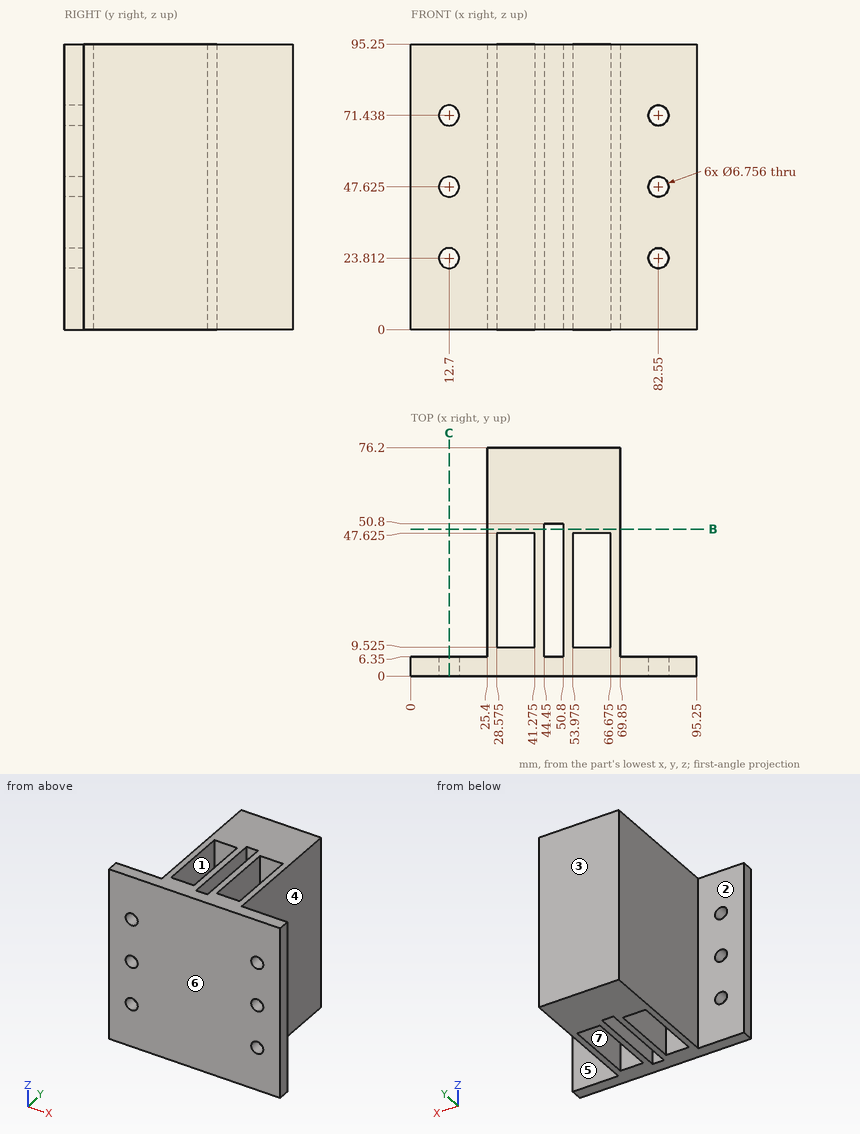
Here's the drawing with two shaded views (mm, measured from the low corner). I have some questions. A direction names the side the tool comes from. Give positions to 0.01 mm unless a question says otherwise; leave off trailing zeros. Order: outer loops, then holes, each group sorted by start corner. A loop starts at its lowest first (then second) coordinate and runs counter-clockwise, first axis right, second up. Notation, with made-up numbers: (-32.75, 84.5) -> (5.25, 84.5) arc R27 cw to (5.25, 101.5) -> close; hole circle Ø11 at (-10.5, 69.5). An arc over 180 degrees is marked (long way). One line per item, written item: value. Start each with the question number.
1. Imagine slicing it at B-B, the plane y = 49. List the corners of the cut face in (x, z) for me.
2. Imagine slicing it at C-C, the plane x = 12.7. Count the separate pieces of the cut face and the enclosed holes in it, plus the area to 3 significant figures.
3. For the marked faces 1, 2, 3 and 4, which set-ups out of +Z, -Z, +X, -X, +Y, -Y let a thin tool reach every point of the face, with its end or its side?
4. I need wall thicknesses on probe 1 along Y at (x, z) = (31.5, 61) (1 decimal); probe 2 along Y at (x, z) = (46.5, 21.5); probe 3 along Z at (x, y) = (12, 3). Which ranges of each line are inside material? Lowest first, please. Write a range as from..to.
5. Will these pins go through, and if not, where does the flat tip stop? pin 1 Ø12.5 at (x, z) = (80.5, 34) entering from +Y; pin 2 Ø11.5 at (y, z) = (28.5, 69.5) entering from +X; pin 3 Ø19 at (y, z) = (29.5, 61) entering from -X; pin 4 Ø4 at (x, z) = (82.55, 71.44) entering from +Y.
6. We'd pull the mould along Y, two halves only. Please class the marked faces 5, 6 and 7: released by +Y, released by -Y, zero draft, split by the parting line, or undercut.
Values follow:
1. outline: (25.4, 0) -> (44.45, 0) -> (44.45, 95.25) -> (25.4, 95.25) -> close; (50.8, 0) -> (69.85, 0) -> (69.85, 95.25) -> (50.8, 95.25) -> close
2. separate pieces: 4
2. enclosed holes: 0
2. area: 476 mm2
3. face 1: +Z, -Z
3. face 2: +Z, -Z, -X, +Y
3. face 3: +Z, -Z, +X, -X, +Y
3. face 4: +Z, -Z, +X, +Y
4. probe 1: y = 0..9.5, 47.6..76.2
4. probe 2: y = 0..6.35, 50.8..76.2
4. probe 3: z = 0..20.51, 27.12..44.32, 50.93..68.13, 74.74..95.25
5. pin 1: stops at y = 6.35
5. pin 2: stops at x = 69.85
5. pin 3: stops at x = 25.4
5. pin 4: passes through
6. face 5: released by +Y
6. face 6: released by -Y
6. face 7: undercut
